```python
from build123d import *

# Parameters (mm, degrees)
SKETCH_1_W          = 12
SKETCH_1_H          = 22
EXTRUDE_1_DEPTH     = 16
SKETCH_2_W          = 12
SKETCH_2_H          = 32
EXTRUDE_2_DEPTH     = 2.5
SKETCH_4_W          = 12
SKETCH_4_H          = 22
EXTRUDE_4_DEPTH     = 5
SKETCH_5_RX         = 7.637200615
SKETCH_5_RY         = 6
EXTRUDE_5_DEPTH     = 5
SKETCH_6_R          = 2.5
EXTRUDE_6_DEPTH     = 3
SKETCH_7_W          = 5
SKETCH_7_H          = 2.5
CUT_EXTRUDE_1_DEPTH = 38.312866414


with BuildPart() as part:
    # 草图1 → 凸台-拉伸1 (new body)
    with BuildSketch(Plane(origin=(0, 0, 0), x_dir=(1, 0, 0), z_dir=(0, 1, 0))):
        Rectangle(SKETCH_1_W, SKETCH_1_H)
    extrude(amount=EXTRUDE_1_DEPTH)

    # 草图2 → 凸台-拉伸2 (add)
    with BuildSketch(Plane(origin=(0, 16, 0), x_dir=(1, 0, 0), z_dir=(0, 1, 0))):
        Rectangle(SKETCH_2_W, SKETCH_2_H)
    extrude(amount=EXTRUDE_2_DEPTH)

    # 草图4 → 凸台-拉伸4 (add)
    with BuildSketch(Plane(origin=(0, 18.5, 0), x_dir=(1, 0, 0), z_dir=(0, 1, 0))):
        Rectangle(SKETCH_4_W, SKETCH_4_H)
    extrude(amount=EXTRUDE_4_DEPTH)

    # 草图5 → 凸台-拉伸5 (add)
    with BuildSketch(Plane(origin=(0, 23.5, 0), x_dir=(1, 0, 0), z_dir=(0, 1, 0))):
        with Locations(Location((0, -3.362799385), (0, 0, -90))):
            Ellipse(SKETCH_5_RX, SKETCH_5_RY)
    extrude(amount=EXTRUDE_5_DEPTH)

    # 草图6 → 凸台-拉伸6 (add)
    with BuildSketch(Plane(origin=(0, 28.5, 0), x_dir=(1, 0, 0), z_dir=(0, 1, 0))):
        with Locations(Location((0, -3.362799385, 0), (0, 0, 270))):
            Circle(SKETCH_6_R)
    extrude(amount=EXTRUDE_6_DEPTH)

    # 草图7 → 切除-拉伸1 (cut, through all)
    with BuildSketch(Plane.ZY.offset(6)):
        with Locations((-13.5, 17.25)):
            Rectangle(SKETCH_7_W, SKETCH_7_H)
        with Locations((13.5, 17.25)):
            Rectangle(SKETCH_7_W, SKETCH_7_H)
    extrude(amount=-CUT_EXTRUDE_1_DEPTH, mode=Mode.SUBTRACT)


solid = part.part
```
Work out the finished part from the listing and answer in its coordinate system (mm). A direction names the side the tool comes from. Give positions to 0.01 mm unless a question says otherwise; leave off trailing zeros. Answer as CSV lines item,"result". Start each with the question number.
(1) Each of these flat-tipped pins is pushed along its axis until it touches: pin 1 Ø1 at (x, z) = (0.5, -9) entering from +Y; pin 2 Ø1.8 at (x, z) = (-3.5, 8.5) entering from +Y. Where does it stop, or does it pass through?
(2) Which of the six approach directions +Z, -Z, +X, -X, +Y, -Y give full straight-line access (tool end or side, diameter ignored) to faces 1 (the flat face through (-5, 23.5, 9)), 2 (the cylindrical face through (0.751, 29.979, 5.747)), 3 (the flat face through (5, 23.5, 9))?
(3) Consider line 1 along Y through (x, z) = (5, 4.25); line 2 along Y through (x, z) = (-3.75, -9.5); line 3 along Z through (x, y) = (-1.25, 27). Determine where each line is inside the solid, lowest interval first.
Entries:
1,pin 1,"y = 23.5"
1,pin 2,"y = 28.5"
2,face 1,"+Z, -X, +Y"
2,face 2,"+Y"
2,face 3,"+Z, +X, +Y"
3,line 1,"0 to 28.5"
3,line 2,"0 to 23.5"
3,line 3,"-4.11 to 10.83"
